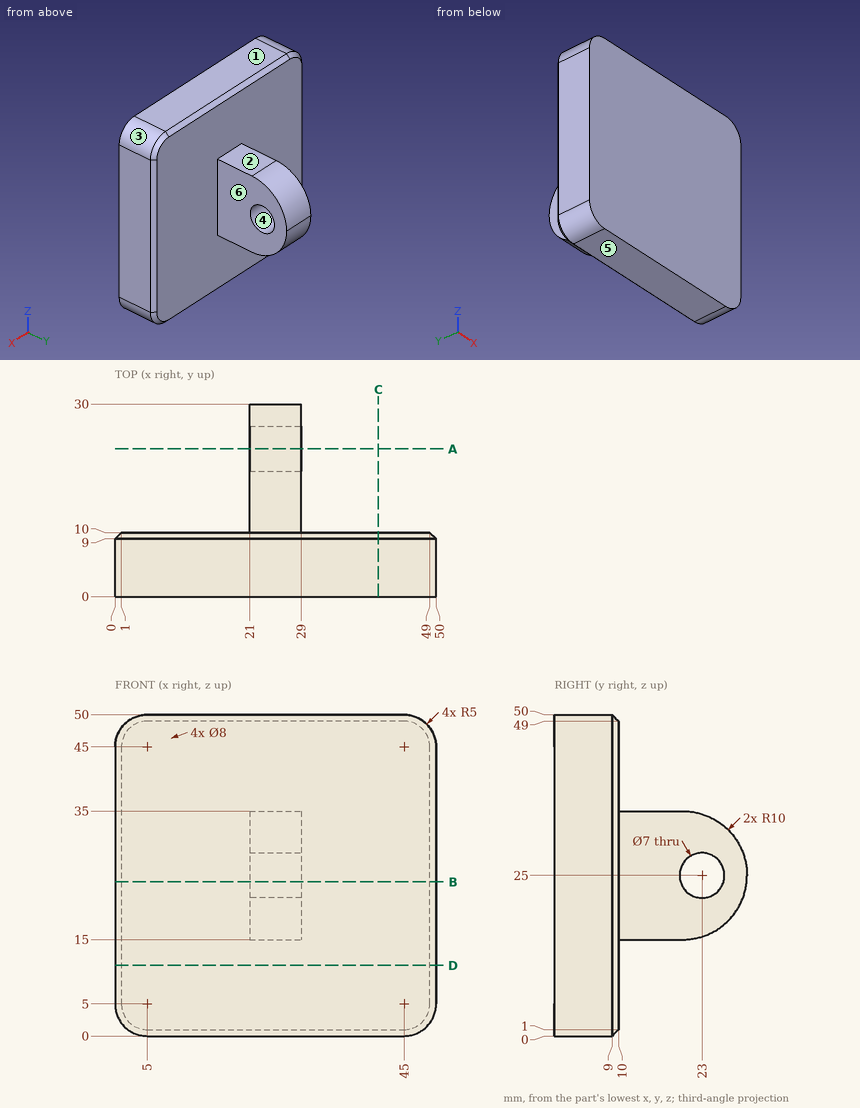
Could you check a few things on this drawing? It's one solid part, dimensions in mm from its lowest x, y, z. A direction names the side the tool comes from. Round coordinates to 2 decimals unless told otherwise and drop trailing zeros. Order: outer loops, then holes, each group sorted by start corner. A loop starts at its lowest first (then second) coordinate and runs counter-clockwise, first axis right, second up. Notation, with made-up numbers: M -31.5,27 L -20.5,27 A26 cw -20.5,57 Z; hole C 76,27 d9. An arc over 180 degrees is marked long. One line per question, with ' | ' between items. Start each with the question number.
(1) Please list where these lines run through material, in increasing order: line 1 along Y through (x, z) = (23, 25); line 2 along Z through (x, y) = (26.5, 22); line 3 along Y through (x, z) = (2, 31).
(2) Suppose I cut it at A-A on y = 23. List the corners of the cut face in (x, z) for me, then the cut area to 3 significant figures.
(3) Suppose I cut it at C-C on x = 41. List the corners of the cut face in (y, z) for me, then the cut area to 3 significant figures.
(4) Suppose I cut it at D-D on z = 11. List the corners of the cut face in (x, y) for me, then the cut area to 3 significant figures.
(5) Suppose I cut it at B-B on z = 24. List the corners of the cut face in (x, y) for me.
(6) Thinking about a two-plate mould opening in Z: for the marked faces 3, 4, 5 and 6, which applies, +Z half, -Z half, draft (parallel to the pull), parting line (faces both ways), or undercut?
(7) For the marked faces 1 and 2, which set-ups out of +Z, -Z, +X, -X, +Y, -Y let a thin tool reach every point of the face, with its end or its side?
(8) For P1, Ø3, axis at y = 16, z = 23, coming from the +X side; P2, Ø6, axis at y = 16.5, z = 40.5, coming from the -X side; P3, Ø2.5, axis at x = 26.5, y = 17, coming from the +Z side; P4, Ø8, axis at x = 33.5, z = 11, coming from the +Y side, each with a flat end and sliding along its axis, tell me the tip position at first contact or that it passes through.
Geometry results:
1) line 1: 0 to 19.5, 26.5 to 30 | line 2: 15.2 to 21.65, 28.35 to 34.8 | line 3: 0 to 10
2) outline: M 21,15.46 L 29,15.46 L 29,21.5 L 21,21.5 Z; M 21,28.5 L 29,28.5 L 29,34.54 L 21,34.54 Z | area: 96.6 mm²
3) outline: M 0,0 L 9,0 L 10,1 L 10,49 L 9,50 L 0,50 Z | area: 499 mm²
4) outline: M 0,0 L 50,0 L 50,9 L 49,10 L 1,10 L 0,9 Z | area: 499 mm²
5) outline: M 0,0 L 50,0 L 50,9 L 49,10 L 29,10 L 29,19.65 L 21,19.65 L 21,10 L 1,10 L 0,9 Z; M 21,26.35 L 29,26.35 L 29,29.95 L 21,29.95 Z
6) face 3: +Z half | face 4: undercut | face 5: -Z half | face 6: draft
7) face 1: +Z, +X, -X, +Y, -Y | face 2: +Z, +X, -X, +Y
8) P1: x = 29 | P2: through | P3: z = 35 | P4: y = 10
